Geometry check sheet. Reference: the model listing, model coordinates, mm. A direction names the side the tool comes from. Coordinates: 2 decimals unless noted, no trailing zeros. Order: outer loops, then holes, each group sorted by start corner. A loop starts at its lowest first (then second) coordinate and runs counter-clockwise, first axis right, second up. Notation, with made-up numbers: (82, 78) - (136, 78) arc R23 ccw to (136, 96) - close; hole circle Ø4 at (12, 64.5). An arc over 180 degrees is marked (long way). Use CSV: the item, a comma, the result in double quotes. Start each with the question number.
1) Depth check by flat-ended pin: P1, Ø12, axis at x = 94, y = -8, coming from the -Z side. Enter the tip coordinate at first touch or a pass-through.
2) Thickness scan on probe 1 along Z at (x, y) = (94, -15.75); probe 2 along X at (y, z) = (-18.75, -138); probe 3 along Z at (x, y) = (59, -5). Record the ranges inside material, lowest first. Write a range as [from, to].
3) Tool access check on faces 1 (the flat face through (142, -13, -130)), 2 (the flat face through (200, -12, 8)). Record the directions out of +Z, -Z, +X, -X, +Y, -Y that give a thin tool (end or side, any length) a straight path to the whole face; none if there is none.
4) Sectioned sample at A-A, the plane y = -15. Record the cut outline in (x, z), and give its area (3 significant figures).
from build123d import *

# Parameters (mm, degrees)
F0_W     = 400
F0_H     = 300
F1_DEPTH = 25
F3_DEPTH = 25.001
F4_R     = 2


with BuildPart() as f1:
    # F0 (on Front) → F1 (new body)
    with BuildSketch(Plane.XZ):
        Rectangle(F0_W, F0_H)
    extrude(amount=F1_DEPTH)

    # F2 (on face) → F3 (cut, through all)
    with BuildSketch(Plane.XZ.offset(25)):
        Polygon((84.6410161514, -130), (50, -150), (200, -150), (200, -130), align=None)
    extrude(amount=-F3_DEPTH, mode=Mode.SUBTRACT)

    # F4
    f4_edges = [f1.edges().sort_by_distance(p)[0] for p in [
        (200, -12.5, 150),
        (200, -12.5, -130),
        (-200, -12.5, -150),
        (-200, -12.5, 150),
        (50, -12.5, -150),
        (84.641016, -12.5, -130),
    ]]
    fillet(f4_edges, radius=F4_R)


solid = f1.part
Evaluation:
1,P1,"z = -130"
2,probe 1,"[-130, 150]"
2,probe 2,"[-200, 70.78]"
2,probe 3,"[-144.8, 150]"
3,face 1,"-Z, +X, +Y, -Y"
3,face 2,"+Z, -Z, +X, +Y, -Y"
4,outline,"(-200, -148) arc R2 ccw to (-198, -150) - (49.46, -150) arc R2 ccw to (50.46, -149.73) - (84.18, -130.27) arc R2 cw to (85.18, -130) - (198, -130) arc R2 ccw to (200, -128) - (200, 148) arc R2 ccw to (198, 150) - (-198, 150) arc R2 ccw to (-200, 148) - close"
4,area,"117,000 mm²"
